from build123d import *

# Parameters (mm, degrees)
SKETCH1_W           = 25
SKETCH1_H           = 24
SKETCH1_R           = 1
BOSS_EXTRUDE1_DEPTH = 1
SKETCH2_W           = 11
SKETCH2_H           = 11
BOSS_EXTRUDE2_DEPTH = 4
SKETCH3_R           = 1.853795749
BOSS_EXTRUDE3_DEPTH = 2


with BuildPart() as part:
    # Sketch1 → Boss-Extrude1 (new body)
    with BuildSketch(Plane.XY):
        with Locations((12.5, 12)):
            Rectangle(SKETCH1_W, SKETCH1_H)
        with Locations((2, 2)):
            Circle(SKETCH1_R, mode=Mode.SUBTRACT)
        with Locations((23, 2)):
            Circle(SKETCH1_R, mode=Mode.SUBTRACT)
        with Locations((2, 14.5)):
            Circle(SKETCH1_R, mode=Mode.SUBTRACT)
        with Locations((23, 14.5)):
            Circle(SKETCH1_R, mode=Mode.SUBTRACT)
    extrude(amount=BOSS_EXTRUDE1_DEPTH)

    # Sketch2 → Boss-Extrude2 (add)
    with BuildSketch(Plane.XY.offset(1)):
        with Locations((12.5, 14.5)):
            Rectangle(SKETCH2_W, SKETCH2_H)
    extrude(amount=BOSS_EXTRUDE2_DEPTH)

    # Sketch3 → Boss-Extrude3 (add)
    with BuildSketch(Plane.XY.offset(5)):
        with Locations((12.5, 14.5)):
            Circle(SKETCH3_R)
    extrude(amount=BOSS_EXTRUDE3_DEPTH)


solid = part.part
Design review of the part built by this model. Coordinates are the model's own, in mm. A direction names the side the tool comes from. Give positions to 0.01 mm unless a question says otherwise; leave off trailing zeros. Order: outer loops, then holes, each group sorted by start corner. A loop starts at its lowest first (then second) coordinate and runs counter-clockwise, first axis right, second up.
1. Add section B-B, the plane x = 2. State the section outline as (y, z) points, then the cut area to 3 significant figures.
Solution:
outline: (0, 0) - (1, 0) - (1, 1) - (0, 1) - close; (3, 0) - (13.5, 0) - (13.5, 1) - (3, 1) - close; (15.5, 0) - (24, 0) - (24, 1) - (15.5, 1) - close
area: 20.0 mm2
2. Mouldability with a two-part tool opening along X and no side actions: class faces 1 (the cylindrical face through (1.2, 1.4, 0.5)), 2 (the flat face through (18, 14, 3)), 3 (the flat face through (12, 12, 0)) as +X half, -X half, draft (parallel to the pull), parting line (faces both ways), or undercut.
Solution:
face 1: undercut
face 2: +X half
face 3: draft
3. Tool access review of faces 4 (the flat face through (12, 20, 3)), 5 (the flat face through (12, 9, 3)), 6 (the flat face through (7, 14, 3)), 7 (the cylindrical face through (10.648, 14.582, 5.986)): name each direction out of +Z, -Z, +X, -X, +Y, -Y from which nothing blocks a thin tool from reaching the whole face with its end or side.
Solution:
face 4: +Z, +X, -X, +Y
face 5: +Z, +X, -X, -Y
face 6: +Z, -X, +Y, -Y
face 7: +Z
4. For pin 1 Ø3 at (x, z) = (11.5, 3.5) entering from -Y; pin 2 Ø10 at (x, y) = (7.5, 4.5) entering from +Z; pin 3 Ø9 at (x, y) = (14, 16.5) entering from +Z; pin 4 Ø2 at (x, z) = (12, 3.5) entering from +Y, all flat-tipped, find the tip position at first contact; note any pin that passes through.
Solution:
pin 1: stops at y = 9
pin 2: stops at z = 5
pin 3: stops at z = 7
pin 4: stops at y = 20
5. To check wall thickness, follow L1, parallel to Y at x = 2, z = 0.35; L2, parallel to Y at x = 7.5, z = 2.25; L3, parallel to Z at x = 24, y = 5.75. State the ranges of each line that lie inside material, in increasing order.
Solution:
L1: y = 0 to 1, 3 to 13.5, 15.5 to 24
L2: y = 9 to 20
L3: z = 0 to 1
6. Add section C-C, the plane y = 17. State the section outline as (x, z) points, then the cut area to 3 significant figures.
Solution:
outline: (0, 0) - (25, 0) - (25, 1) - (18, 1) - (18, 5) - (7, 5) - (7, 1) - (0, 1) - close
area: 69.0 mm2
7. Add section A-A, the plane y = 2. State the section outline as (x, z) points.
Solution:
outline: (0, 0) - (1, 0) - (1, 1) - (0, 1) - close; (3, 0) - (22, 0) - (22, 1) - (3, 1) - close; (24, 0) - (25, 0) - (25, 1) - (24, 1) - close
8. Add section D-D, the plane x = 9.5. State the section outline as (y, z) points.
Solution:
outline: (0, 0) - (24, 0) - (24, 1) - (20, 1) - (20, 5) - (9, 5) - (9, 1) - (0, 1) - close
